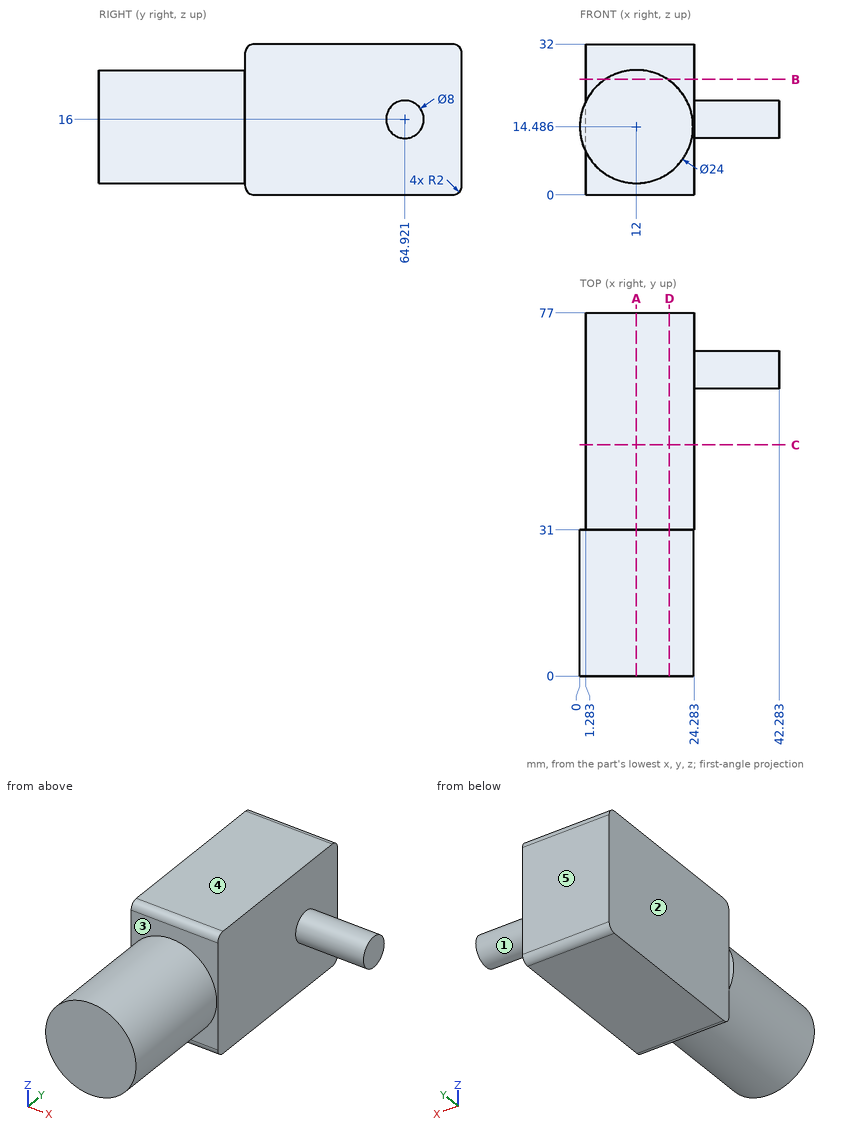
Print and shaded views of the part. All mm, measured from the part's lowest x, y and z. A direction names the side the tool comes from. Give positions to 0.01 mm unless a question says otherwise; leave off trailing zeros. Loops run counter-clockwise (first coordinate to the right, second up) from the corner with the lowest first, then second, coordinate; pieces in that order, holes last. Notation, with made-up numbers: (81.25, 15) -> (139.25, 15) arc R15 cw to (139.25, 44) -> close; hole circle Ø7 at (60, 31). An arc over 180 degrees is marked (long way). Answer in a Markdown table with one row per item.
Item 1: Flat gauge pins, fed straight in: P1, Ø10, axis at y = 67.5, z = 20, coming from the -X side; P2, Ø1, axis at y = 44, z = 3.5, coming from the +X side; P3, Ø3, axis at y = 29, z = 9, coming from the +X side. Where does each tip first touch, or does it go through?
Findings below:
| item | result |
|---|---|
| P1 | stops at x = 1.28 |
| P2 | stops at x = 24.28 |
| P3 | stops at x = 23.32 |
Item 2: Slice it at C-C on y = 49. Write the cut outline in (x, z).
Findings below:
| item | result |
|---|---|
| outline | (1.28, 0) -> (24.28, 0) -> (24.28, 32) -> (1.28, 32) -> close |
Item 3: Slice it at A-A on x = 12. Write the cut outline in (y, z).
Findings below:
| item | result |
|---|---|
| outline | (0, 2.49) -> (31, 2.49) -> (31, 2) arc R2 ccw to (33, 0) -> (75, 0) arc R2 ccw to (77, 2) -> (77, 30) arc R2 ccw to (75, 32) -> (33, 32) arc R2 ccw to (31, 30) -> (31, 26.49) -> (0, 26.49) -> close |
Item 4: Probe line 1 along X through (y, z) = (53, 13); line 2 along X through (y, z) = (65, 14.5); line 3 along Y through (x, z) = (9, 29.5). List the from-to ranges inside material, lowest first. Write a range as [from, to].
Findings below:
| item | result |
|---|---|
| line 1 | x = [1.28, 24.28] |
| line 2 | x = [1.28, 42.28] |
| line 3 | y = [31, 77] |
Item 5: Slice it at D-D on x = 19. Write the cut outline in (y, z), plus the area to 3 significant figures.
Findings below:
| item | result |
|---|---|
| outline | (0, 4.74) -> (31, 4.74) -> (31, 2) arc R2 ccw to (33, 0) -> (75, 0) arc R2 ccw to (77, 2) -> (77, 30) arc R2 ccw to (75, 32) -> (33, 32) arc R2 ccw to (31, 30) -> (31, 24.23) -> (0, 24.23) -> close |
| area | 2,070 mm² |
Item 6: Slice it at B-B on z = 24.5. Write the cut outline in (x, y), plus the area to 3 significant figures.
Findings below:
| item | result |
|---|---|
| outline | (1.28, 31) -> (5.39, 31) -> (5.39, 0) -> (18.61, 0) -> (18.61, 31) -> (24.28, 31) -> (24.28, 77) -> (1.28, 77) -> close |
| area | 1,470 mm² |
Item 7: Tool access for the marked faces 1, 2, 3, 4 and 5: list every direction of +Z, -Z, +X, -X, +Y, -Y with a clear straight run to the whole face (end or side of a thin tool).
Findings below:
| item | result |
|---|---|
| face 1 | +X |
| face 2 | +Z, -Z, -X, +Y |
| face 3 | -Y |
| face 4 | +Z, +X, -X, +Y, -Y |
| face 5 | +Z, -Z, +X, -X, +Y |
